```python
from build123d import *

# Parameters (mm, degrees)
SKETCH1_W               = 1524
SKETCH1_H               = 762
BOSS_EXTRUDE1_DEPTH     = 31.75
SKETCH2_W               = 50.8
SKETCH2_H               = 50.8
BOSS_EXTRUDE2_DEPTH     = 584.2
SKETCH3_R               = 12.7
BOSS_EXTRUDE3_DEPTH     = 101.6
SKETCH4_R               = 63.5
BOSS_EXTRUDE4_DEPTH     = 14.2875
MIRROR2_COPY_1_SKETCH_R = 63.5
MIRROR2_COPY_1_DEPTH    = 14.2875


with BuildPart() as part:
    # Sketch1 → Boss-Extrude1 (new body)
    with BuildSketch(Plane(origin=(0, 0, 0), x_dir=(1, 0, 0), z_dir=(0, 1, 0))):
        Rectangle(SKETCH1_W, SKETCH1_H)
    extrude(amount=-BOSS_EXTRUDE1_DEPTH)

    # Sketch2 → Boss-Extrude2 (add)
    with BuildSketch(Plane.XZ.offset(31.75)):
        with Locations((-711.2, 330.2)):
            Rectangle(SKETCH2_W, SKETCH2_H)
        with Locations((-711.2, -330.2)):
            Rectangle(SKETCH2_W, SKETCH2_H)
        with Locations((711.2, -330.2)):
            Rectangle(SKETCH2_W, SKETCH2_H)
        with Locations((711.2, 330.2)):
            Rectangle(SKETCH2_W, SKETCH2_H)
    extrude(amount=BOSS_EXTRUDE2_DEPTH)

    # Sketch3 → Boss-Extrude3 (add)
    with BuildSketch(Plane.XZ.offset(615.95)):
        with Locations(Location((711.2, 330.2, 0), (0, 0, 270))):
            Circle(SKETCH3_R)
        with Locations(Location((711.2, -330.2, 0), (0, 0, 270))):
            Circle(SKETCH3_R)
        with Locations(Location((-711.2, -330.2, 0), (0, 0, 270))):
            Circle(SKETCH3_R)
        with Locations(Location((-711.2, 330.2, 0), (0, 0, 270))):
            Circle(SKETCH3_R)
    extrude(amount=BOSS_EXTRUDE3_DEPTH)

    # Sketch4 → Boss-Extrude4 (add, symmetric)
    with BuildSketch(Plane(origin=(0, 0, 0), x_dir=(0.9070089677484316, 0, 0.42111130645462913), z_dir=(-0.4211113064546291, 0, 0.9070089677484315))):
        with Locations((752.365731254, -698.5)):
            Circle(SKETCH4_R)
    boss_extrude4 = extrude(amount=BOSS_EXTRUDE4_DEPTH, both=True)

    # Mirror1: Boss-Extrude4 across plane
    add(boss_extrude4.mirror(Plane.XY))

    # Mirror2: Boss-Extrude4 across plane
    add(boss_extrude4.mirror(Plane(origin=(0, 0, 0), x_dir=(0, 0, 1), z_dir=(1, 0, 0))))

    # Mirror2 copy 1 sketch → Mirror2 copy 1 (add, symmetric)
    with BuildSketch(Plane(origin=(0, 0, 0), x_dir=(-0.9070089677484316, 0, -0.42111130645462913), z_dir=(0.4211113064546291, 0, -0.9070089677484315))):
        with Locations((752.365731254, -698.5)):
            Circle(MIRROR2_COPY_1_SKETCH_R)
    extrude(amount=MIRROR2_COPY_1_DEPTH, both=True)


solid = part.part
```
Source: CAD feature listing. Evaluate the final solid. Frame: model axes, mm. A direction names the side the tool comes from. Round coordinates to 2 decimals unless told otherwise and drop trailing zeros. Loops run counter-clockwise (first coordinate to the right, second up) from the corner with the lowest first, then second, coordinate; pieces in that order, holes last. Notation, with made-up numbers: M -23.5,-8 L -16.5,-8 A21 cw -16.5,13 Z; hole C 19.5,81 d8. An arc over 180 degrees is marked long. Use a Markdown table: item, result. Add a question column.
1. Section query D-D on y = -671.5. Return the cut outline in (x, z).
2. Mould query, pull axis Y, two halves, no side actions, for faces 4 (the flat face through (687.613, -697.611, -303.496)), 5 (the flat face through (-11, 0, -5)), 6 (the cylindrical face through (669.83, -760.49, -311.21)). Classes: pulls with the +Y half, pulls with the -Y half, needs draft (parallel to the pull), parting line crosses it, or undercut.
3. Section query A-A on y = -279. Return the cut outline in (x, z), then the cut area to 3 significant figures.
4. Section query B-B on x = 520. Return the cut outline in (y, z), then the cut area to 3 significant figures.
5. Line query: line 1 (Z direction, x = -686.5, y = -568); line 2 (X direction, y = -238, z = 319); line 3 (Y direction, x = 159.5, z = 67.5). Output: solid intervals per line, ascending.
6. Reachability of faces 1 (the flat face through (705, -615.95, 342)), 2 (the flat face through (-736.6, -320, -331)), 3 (the flat face through (-685.8, -320, -331)) from +Z, -Z, +X, -X, +Y, -Y: full face, straight path, thin tool, end or side. Return the list, or none.
7. Contact query for flat-ended pins moving along their axis: P1, Ø10, axis at x = -157, z = -277, coming from the -Y side; P2, Ø15, axis at y = -261.5, z = -339, coming from the -X side. Output: stop coordinate, or through.
8. Section query C-C on z = 248. Return the cut outline in (x, y).
Reported:
| question | item | result |
|---|---|---|
| 1 | outline | M -740.55,-328.07 L -728.52,-353.99 L -624.26,-305.59 L -636.29,-279.67 Z; M -740.55,328.07 L -636.29,279.67 L -624.26,305.59 L -728.52,353.99 Z; M 624.26,-305.59 L 728.52,-353.99 L 740.55,-328.07 L 636.29,-279.67 Z; M 624.26,305.59 L 636.29,279.67 L 740.55,328.07 L 728.52,353.99 Z |
| 2 | face 4 | needs draft |
| 2 | face 5 | pulls with the +Y half |
| 2 | face 6 | undercut |
| 3 | outline | M -736.6,-355.6 L -685.8,-355.6 L -685.8,-304.8 L -736.6,-304.8 Z; M -736.6,304.8 L -685.8,304.8 L -685.8,355.6 L -736.6,355.6 Z; M 685.8,-355.6 L 736.6,-355.6 L 736.6,-304.8 L 685.8,-304.8 Z; M 685.8,304.8 L 736.6,304.8 L 736.6,355.6 L 685.8,355.6 Z |
| 3 | area | 10,300 mm² |
| 4 | outline | M -31.75,-381 L 0,-381 L 0,381 L -31.75,381 Z |
| 4 | area | 24,200 mm² |
| 5 | line 1 | z = -355.6 to -304.8, 304.8 to 355.6 |
| 5 | line 2 | x = -736.6 to -685.8, 685.8 to 736.6 |
| 5 | line 3 | y = -31.75 to 0 |
| 6 | face 1 | none |
| 6 | face 2 | +Z, -Z, -X |
| 6 | face 3 | +Z, -Z |
| 7 | P1 | stops at y = -31.75 |
| 7 | P2 | stops at x = -736.6 |
| 8 | outline | M -762,-31.75 L 762,-31.75 L 762,0 L -762,0 Z |
